Input: part model. Units: mm. Frame: model coordinates. A direction names the side the tool comes from. Give positions to 0.01 mm unless a question says otherwise; leave off trailing zeros. Loops run counter-clockwise (first coordinate to the right, second up) from the corner with the lowest first, then second, coordinate; pieces in that order, holes last. Notation, with made-up numbers: (-35.75, 5) -> (5.25, 5) arc R27 ccw to (5.25, 36) -> close; hole circle Ø7 at (-17.5, -34.75). An arc over 180 degrees is marked (long way). One line per question, with ' | ' between items.
Autodesk Inventor part; units mm, degrees
ref_plane "YZ Plane" through (0, 0, 0) normal (1, 0, 0) x (0, 1, 0)
ref_plane "XZ Plane" through (0, 0, 0) normal (0, 1, 0) x (-1, 0, 0)
ref_plane "XY Plane" through (0, 0, 0) normal (0, 0, 1) x (1, 0, 0)
sketch "Sketch1" plane through (0, 0, 0) normal (0, 1, 0) x (-1, 0, 0)
  line L0 (-42, 2.5) -> (42, 2.5)
  line L1 (42, 2.5) -> (42, -2.5)
  line L2 (42, -2.5) -> (-42, -2.5)
  line L3 (-42, -2.5) -> (-42, 2.5)
  line L4 (-42, 2.5) -> (42, -2.5) construction
  line L5 (42, 2.5) -> (-42, -2.5) construction
  point P0 (0, 0)
  dimension "d0" = 84
  dimension "d1" = 5
extrude "Extrusion1" add sketch "Sketch1" along normal blind 4
sketch "Sketch2" plane through (0, 4, 0) normal (0, 1, 0) x (1, 0, 0)
  circle A0 centre (-37, 0) radius 1.25
  circle A1 centre (37, 0) radius 1.25
  line L0 (42, -2.5) -> (42, 2.5)
  line L1 (-42, -2.5) -> (-42, 2.5)
  point P0 (0, 0)
  dimension "d4" = 2.5
  dimension "d5" = 2.5
  dimension "d6" = 5
  dimension "d7" = 5
extrude "Extrusion2" cut sketch "Sketch2" against normal up to next
sketch "Sketch3" plane through (-42, 0, 2.5) normal (0, 0, 1) x (1, 0, 0)
  line L0 (84, 4) -> (0, 4)
  line L1 (0, 4) -> (84, 4)
  line L2 (84, 4) -> (84, 0)
  line L3 (84, 0) -> (0, 0)
  line L4 (0, 0) -> (0, 4)
  point P0 (42, 0)
extrude "Extrusion3" add sketch "Sketch3" along normal blind 3
sketch "Sketch4" plane through (-42, 0, 5.5) normal (0, 0, 1) x (1, 0, 0)
  line L0 (84, 4) -> (70, 4)
  line L1 (84, 4) -> (0, 4)
  line L2 (0, 4) -> (14, 4)
  line L3 (14, 4) -> (21, 4)
  line L4 (21, 4) -> (21, -2)
  line L5 (21, -2) -> (14, -2)
  line L6 (14, -2) -> (14, 4)
  line L7 (70, 4) -> (63, 4)
  line L8 (63, 4) -> (63, -2)
  line L9 (63, -2) -> (70, -2)
  line L10 (70, -2) -> (70, 4)
  point P0 (42, 0)
  dimension "d12" = 14
  dimension "d13" = 14
  dimension "d14" = 7
  dimension "d15" = 6
  dimension "d16" = 7
  dimension "d17" = 6
extrude "Extrusion4" add sketch "Sketch4" along normal blind 6
sketch "Sketch5" plane through (28, -2, 5.5) normal (1, 0, 0) x (0, 0, -1)
  line L0 (0, 6) -> (-6, 3.8162)
  line L1 (-6, 0) -> (-6, 6)
  line L2 (0, 6) -> (6.3851, 6) construction
  line L3 (-6, 3.8162) -> (-6, 6)
  line L4 (0, 6) -> (-6, 6)
  line L5 (0, 6) -> (-6, 6)
  point P0 (5.5, 2)
  dimension "d20" = 160
extrude "Extrusion5" cut sketch "Sketch5" against normal through all
sketch "Sketch6" plane through (28, -2, 5.5) normal (1, 0, 0) x (0, 0, -1)
  line L0 (0, 0) -> (0, 2)
  line L1 (0, 0) -> (-6, 0)
  line L2 (0, 2) -> (-6, 0)
  point P0 (5.5, 2)
extrude "Extrusion6" cut sketch "Sketch6" against normal through all
sketch "Sketch7" plane through (21, 1.8162, 11.5) normal (0, 0.9397, 0.342) x (1, 0, 0)
  line L0 (0, -1.3052) -> (7, -1.3052)
  line L1 (3.5, -1.3052) -> (3.5, 3.6948)
  circle A0 centre (3.5, 3.6948) radius 1.25
  line L2 (-49, -1.3052) -> (-42, -1.3052)
  line L3 (-45.5, -1.3052) -> (-45.5, 3.6948)
  circle A1 centre (-45.5, 3.6948) radius 1.25
  point P0 (-21, 10.1853)
  dimension "d25" = 5
  dimension "d26" = 2.5
  dimension "d27" = 5
  dimension "d28" = 2.5
extrude "Extrusion7" cut sketch "Sketch7" against normal up to next
properties part number "rpi_stabilizer"
1. Section query C-C (x = -27). Output: boundary loops of the cut face in (y, z).
Determined:
outline: (-2, 11.5) -> (0, 5.5) -> (0, -2.5) -> (4, -2.5) -> (4, 5.5) -> (1.82, 11.5) -> close
2. Section query B-B (z = 0). Output: boundary loops of the cut face in (x, y), then the cut area to 3 significant figures.
Determined:
outline: (-42, 0) -> (-38.25, 0) -> (-38.25, 4) -> (-42, 4) -> close; (-35.75, 0) -> (35.75, 0) -> (35.75, 4) -> (-35.75, 4) -> close; (38.25, 0) -> (42, 0) -> (42, 4) -> (38.25, 4) -> close | area: 316 mm2
3. Section query D-D (z = 3.5). Output: boundary loops of the cut face in (x, y), then the cut area to 3 significant figures.
Determined:
outline: (-42, 0) -> (42, 0) -> (42, 4) -> (-42, 4) -> close | area: 336 mm2
4. Reachability of faces 4 (the flat face through (28, 1, 8)), 5 (the flat face through (21, 1, 8)), 6 (the flat face through (-24.5, -1, 8.5)) from +Z, -Z, +X, -X, +Y, -Y: full face, straight path, thin tool, end or side. Return the list, or none.
Determined:
face 4: +Z, +X, +Y, -Y | face 5: +Z, +Y, -Y | face 6: -Z, +X, -X, -Y
5. Section query A-A (x = 37). Output: boundary loops of the cut face in (y, z).
Determined:
outline: (0, -2.5) -> (4, -2.5) -> (4, -1.25) -> (0, -1.25) -> close; (0, 1.25) -> (4, 1.25) -> (4, 5.5) -> (0, 5.5) -> close
6. Pull-direction query (Y, two-part tool) for faces 1 (the flat face through (25.327, 2.681, 9.125)), 2 (the flat face through (-28, 1, 8)), 3 (the cylindrical face through (-23.31, 1.47, 7.04)); classes: pulls with the +Y half, pulls with the -Y half, needs draft (parallel to the pull), parting line crosses it, or undercut.
Determined:
face 1: pulls with the +Y half | face 2: needs draft | face 3: undercut
7. Pin query (flat end, axial travel): P1, Ø2, axis at x = 5, z = 7.5, coming from the -Y side; P2, Ø1.2, axis at x = 35.5, y = 1.5, coming from the +Z side; P3, Ø8, axis at x = 14.5, z = 7.5, coming from the -Y side; P4, Ø1.8, axis at y = 2.5, z = 9.5, coming from the +X side. Return the tip coordinate at first contact, or that it passes through.
Determined:
P1: passes through | P2: stops at z = 5.5 | P3: stops at y = 0 | P4: stops at x = 28
8. Ray query, line 1 along X through (y, z) = (2.75, 0); line 2 along Z through (x, y) = (-37, 0.8); line 3 along Y through (x, z) = (-18.5, 0.25). Return the intervals inside material, ascending. Write a range as from..to.
Determined:
line 1: x = -42..-38.25, -35.75..35.75, 38.25..42 | line 2: z = -2.5..-1.25, 1.25..5.5 | line 3: y = 0..4
